Part model, mm, in its own coordinate system. A direction names the side the tool comes from. Round coordinates to 2 decimals unless told otherwise and drop trailing zeros. Loops run counter-clockwise (first coordinate to the right, second up) from the corner with the lowest first, then second, coordinate; pieces in that order, holes last. Notation, with made-up numbers: M 73,47 L 122,47 A24 cw 122,85 Z; hole C 27.5,28 d7. An arc over 180 degrees is marked long. Put each result on its own line as item: value. Start each with the question number.
1) Slice it at B-B on y = -10.5. Give the cut face in (x, z).
2) Which spindle directions (+Z, -Z, +X, -X, +Y, -Y) get a long thin tool onto all of the face, cutting with end or side? Do faces 1 (the flat face through (170.18, 0, 0)), 2 (the cylindrical face through (183.613, 8.255, -0.067)), 3 (the flat face through (38.1, 0, 0)), 4 (the cylindrical face through (183.613, -8.255, 0.067)). Say none if no direction does.
3) Slice it at A-A on x = 28. Give the cut face in (y, z).
4) Drop flat-ended pins along their axis: pin 1 Ø15 at (x, y) = (186, -0.5) entering from -Z; pin 2 Ø1 at (x, y) = (25.5, -4.5) entering from -Z; pin 3 Ø3 at (x, z) = (132, -1.5) entering from +Y. Give the stop position or say it passes through.
5) Pull direction Y, two halves, no side cores. Call faces 5 (the cylindrical face through (6.261, 2.48, -7.874)), 6 (the flat face through (39.646, 0, 0)), 7 (the cylindrical face through (104, 2.52, -0.33)), 8 (the flat face through (187, 0, 4.533)): +Y half, -Y half, draft (parallel to the pull), parting line (faces both ways), or undercut.
6) Probe line 1 along Z through (x, y) = (107, 0); line 2 along X through (y, z) = (5.25, -6); line 3 along Y through (x, z) = (33, -0.5). List the from-to ranges inside material, lowest first.
```python
from build123d import *

# Parameters (mm, degrees)
CROQUIS2_R                   = 12.7
SALIENTE_EXTRUIR1_DEPTH      = 190.5
CROQUIS3_R                   = 12.7
CROQUIS3_R_2                 = 8.255
CORTAR_EXTRUIR1_DEPTH        = 12.7
CROQUIS4_R                   = 2.54
CORTAR_EXTRUIR2_DEPTH        = 170.18
CROQUIS6_R                   = 12.7
CROQUIS6_R_2                 = 8.255
CORTAR_EXTRUIR6_DEPTH        = 16.51
CORTAR_EXTRUIR8_DEPTH        = 16.51
CROQUIS9_R                   = 3.175
CORTAR_EXTRUIR9_DEPTH        = 16.51
CROQUIS10_W                  = 1.546124295
CROQUIS10_H                  = 25.4
SALIENTE_EXTRUIR2_DEPTH      = 12.7
SALIENTE_EXTRUIR2_DEPTH_BACK = 12.7
CORTAR_EXTRUIR10_DEPTH       = 64.262
CORTAR_EXTRUIR11_DEPTH       = 64.262
CORTAR_EXTRUIR12_DEPTH       = 64.262


with BuildPart() as part:
    # Croquis2 → Saliente-Extruir1 (new body)
    with BuildSketch(Plane(origin=(0, 0, 0), x_dir=(0, 0, -1), z_dir=(1, 0, 0))):
        Circle(CROQUIS2_R)
    extrude(amount=SALIENTE_EXTRUIR1_DEPTH)

    # Croquis3 → Cortar-Extruir1 (cut)
    with BuildSketch(Plane(origin=(0, 0, 0), x_dir=(0, 0, -1), z_dir=(1, 0, 0))):
        Circle(CROQUIS3_R)
        Circle(CROQUIS3_R_2, mode=Mode.SUBTRACT)
    extrude(amount=CORTAR_EXTRUIR1_DEPTH, mode=Mode.SUBTRACT)

    # Croquis4 → Cortar-Extruir2 (cut)
    with BuildSketch(Plane.ZY):
        Circle(CROQUIS4_R)
    extrude(amount=-CORTAR_EXTRUIR2_DEPTH, mode=Mode.SUBTRACT)

    # Croquis6 → Cortar-Extruir6 (cut)
    with BuildSketch(Plane(origin=(193.04, 0, 0), x_dir=(0, 0, -1), z_dir=(1, 0, 0))):
        Circle(CROQUIS6_R)
        Circle(CROQUIS6_R_2, mode=Mode.SUBTRACT)
    extrude(amount=-CORTAR_EXTRUIR6_DEPTH, mode=Mode.SUBTRACT)

    # Croquis8 → Cortar-Extruir8 (cut)
    with BuildSketch(Plane(origin=(193.04, 0, 0), x_dir=(0, 0, -1), z_dir=(1, 0, 0))):
        with BuildLine():
            Line((-4.533022208, 6.899038677), (-4.533022208, -6.899038677))
            ThreePointArc((-4.533022208, -6.899038677), (-8.255, 0), (-4.533022208, 6.899038677))
        make_face()
        with BuildLine():
            Line((4.533022208, 6.899038677), (4.533022208, -6.899038677))
            ThreePointArc((4.533022208, -6.899038677), (8.255, 0), (4.533022208, 6.899038677))
        make_face()
    extrude(amount=-CORTAR_EXTRUIR8_DEPTH, mode=Mode.SUBTRACT)

    # Croquis9 → Cortar-Extruir9 (cut)
    with BuildSketch(Plane(origin=(0, 0, -4.533022208), x_dir=(-1, 0, 0), z_dir=(0, 0, -1))):
        with Locations((-183.515, 0)):
            Circle(CROQUIS9_R)
    extrude(amount=-CORTAR_EXTRUIR9_DEPTH, mode=Mode.SUBTRACT)

    # Croquis10 → Saliente-Extruir2 (add, two sides)
    with BuildSketch(Plane.XY) as saliente_extruir2_sk:
        with Locations((38.873062148, 0.259017105)):
            Rectangle(CROQUIS10_W, CROQUIS10_H)
    extrude(amount=SALIENTE_EXTRUIR2_DEPTH)
    extrude(saliente_extruir2_sk.sketch, amount=-SALIENTE_EXTRUIR2_DEPTH_BACK)

    # Croquis12 → Cortar-Extruir10 (cut)
    with BuildSketch(Plane(origin=(0, 0, 0), x_dir=(0, 0, -1), z_dir=(1, 0, 0))):
        with BuildLine():
            Line((0, 12.959017105), (-12.7, 12.959017105))
            Line((-12.7, 12.959017105), (-12.7, 2.578007822))
            ThreePointArc((-12.7, 2.578007822), (-8.201453434, 10.033557988), (0, 12.959017105))
        make_face()
    extrude(amount=CORTAR_EXTRUIR10_DEPTH, mode=Mode.SUBTRACT)

    # Croquis13 → Cortar-Extruir11 (cut)
    with BuildSketch(Plane.ZY.offset(-38.1)):
        with BuildLine():
            Line((-12.7, 2.578007822), (-12.7, 12.959017105))
            Line((-12.7, 12.959017105), (0, 12.959017105))
            ThreePointArc((0, 12.959017105), (-8.201453434, 10.033557988), (-12.7, 2.578007822))
        make_face()
    extrude(amount=-CORTAR_EXTRUIR11_DEPTH, mode=Mode.SUBTRACT)

    # Croquis14 → Cortar-Extruir12 (cut)
    with BuildSketch(Plane.ZY.offset(-38.1)):
        with BuildLine():
            Line((12.7, -2.768457402), (12.7, -12.440982895))
            Line((12.7, -12.440982895), (3.765142892, -12.440982895))
            ThreePointArc((3.765142892, -12.440982895), (9.548019164, -8.819846168), (12.7, -2.768457402))
        make_face()
        with BuildLine():
            Line((-12.769462216, -2.428001465), (-12.7, -12.440982895))
            Line((-12.7, -12.440982895), (-3.765142892, -12.440982895))
            ThreePointArc((-3.765142892, -12.440982895), (-9.66505255, -8.691439213), (-12.769462216, -2.428001465))
        make_face()
    extrude(amount=-CORTAR_EXTRUIR12_DEPTH, mode=Mode.SUBTRACT)


solid = part.part
```
Recorded:
1. outline: M 12.7,-7.14 L 38.1,-7.14 L 38.1,-7.66 L 39.65,-7.66 L 39.65,-7.14 L 176.53,-7.14 L 176.53,7.14 L 39.65,7.14 L 39.65,7.66 L 38.1,7.66 L 38.1,7.14 L 12.7,7.14 Z
2. face 1: none
2. face 2: +X, +Y
2. face 3: -X
2. face 4: +X, -Y
3. outline: C 0,0 d25.4; hole C 0,0 d5.08
4. pin 1: stops at z = -4.53
4. pin 2: stops at z = -12.05
4. pin 3: stops at y = 12.7
5. face 5: parting line
5. face 6: undercut
5. face 7: undercut
5. face 8: draft
6. line 1: z = -12.7 to -2.54, 2.54 to 12.7
6. line 2: x = 0 to 176.53
6. line 3: y = -12.69 to -2.49, 2.49 to 12.69
